```python
from build123d import *

# Parameters (mm, degrees)
BOSS_EXTRUDE1_DEPTH   = 3.175
SKETCH2_W             = 12.7
SKETCH2_H             = 12.7
BOSS_EXTRUDE2_DEPTH   = 28.575
SKETCH3_R             = 2.5
CUT_EXTRUDE1_DEPTH    = 10
CHAMFER1_SIZE         = 12.7
CHAMFER1_SIZE2        = 7.332348419
CHAMFER1_PART_2_SIZE  = 12.7
CHAMFER1_PART_2_SIZE2 = 7.332348419
CHAMFER1_PART_3_SIZE  = 12.7
CHAMFER1_PART_3_SIZE2 = 7.332348419
FILLET1_R             = 3.175
FILLET2_R             = 3.175
FILLET4_R             = 1.5875


with BuildPart() as part:
    # Sketch1 → Boss-Extrude1 (new body)
    with BuildSketch(Plane.XY):
        Polygon((38.1, 0), (-38.1, 0), (-38.1, -12.7), (-19.05, -12.7), (-19.05, -69.85), (-6.35, -69.85), (-6.35, -38.1), (19.05, -12.7), (38.1, -12.7), align=None)
    extrude(amount=BOSS_EXTRUDE1_DEPTH)

    # Sketch2 → Boss-Extrude2 (add)
    with BuildSketch(Plane(origin=(0, 0, 0), x_dir=(-1, 0, 0), z_dir=(0, 0, -1))):
        with Locations((-31.75, -6.35)):
            Rectangle(SKETCH2_W, SKETCH2_H)
        with Locations((31.75, -6.35)):
            Rectangle(SKETCH2_W, SKETCH2_H)
        with Locations((12.7, -63.5)):
            Rectangle(SKETCH2_W, SKETCH2_H)
    extrude(amount=BOSS_EXTRUDE2_DEPTH)

    # Sketch3 → Cut-Extrude1 (cut)
    with BuildSketch(Plane(origin=(0, 0, -28.575), x_dir=(-1, 0, 0), z_dir=(0, 0, -1))):
        with Locations((-31.75, -6.35)):
            Circle(SKETCH3_R)
        with Locations((31.75, -6.35)):
            Circle(SKETCH3_R)
        with Locations((12.7, -63.5)):
            Circle(SKETCH3_R)
    extrude(amount=-CUT_EXTRUDE1_DEPTH, mode=Mode.SUBTRACT)

    # Chamfer1
    chamfer1_edges = [part.edges().sort_by_distance(p)[0] for p in [
        (38.1, -6.35, 3.175),
    ]]
    chamfer1_side = [part.faces().sort_by_distance(p)[0] for p in [
        (38.1, -6.35, -12.7),
    ]]
    chamfer(chamfer1_edges, length=CHAMFER1_SIZE, length2=CHAMFER1_SIZE2, reference=chamfer1_side[0])

    # Chamfer1 part 2
    chamfer1_part_2_edges = [part.edges().sort_by_distance(p)[0] for p in [
        (-38.1, -6.35, 3.175),
    ]]
    chamfer1_part_2_side = [part.faces().sort_by_distance(p)[0] for p in [
        (-38.1, -6.35, -12.7),
    ]]
    chamfer(chamfer1_part_2_edges, length=CHAMFER1_PART_2_SIZE, length2=CHAMFER1_PART_2_SIZE2, reference=chamfer1_part_2_side[0])

    # Chamfer1 part 3
    chamfer1_part_3_edges = [part.edges().sort_by_distance(p)[0] for p in [
        (-12.7, -69.85, 3.175),
    ]]
    chamfer1_part_3_side = [part.faces().sort_by_distance(p)[0] for p in [
        (-12.7, -69.85, -12.7),
    ]]
    chamfer(chamfer1_part_3_edges, length=CHAMFER1_PART_3_SIZE, length2=CHAMFER1_PART_3_SIZE2, reference=chamfer1_part_3_side[0])

    # Fillet1
    fillet1_edges = [part.edges().sort_by_distance(p)[0] for p in [
        (-6.35, -38.1, 1.5875),
        (-19.05, -12.7, 1.5875),
        (19.05, -12.7, 1.5875),
    ]]
    fillet(fillet1_edges, radius=FILLET1_R)

    # Fillet2
    fillet2_edges = [part.edges().sort_by_distance(p)[0] for p in [
        (25.4, -12.7, -14.2875),
        (25.4, 0, -14.2875),
        (-25.4, 0, -14.2875),
        (-25.4, -12.7, -14.2875),
        (-19.05, -57.15, -14.2875),
        (-6.35, -57.15, -14.2875),
        (38.1, 0, -19.05),
        (-38.1, 0, -19.05),
        (38.1, -12.7, -19.05),
        (-6.35, -69.85, -19.05),
        (-19.05, -69.85, -19.05),
        (-38.1, -12.7, -19.05),
    ]]
    fillet(fillet2_edges, radius=FILLET2_R)

    # Fillet4
    fillet4_edges = [part.edges().sort_by_distance(p)[0] for p in [
        (-12.7, -57.15, -28.575),
        (-19.05, -63.5, -28.575),
        (-6.35, -63.5, -28.575),
        (-12.7, -69.85, -28.575),
        (-7.27993597, -58.07993597, -28.575),
        (-7.27993597, -68.92006403, -28.575),
        (-18.12006403, -68.92006403, -28.575),
        (-18.12006403, -58.07993597, -28.575),
        (38.1, -6.35, -28.575),
        (31.75, -12.7, -28.575),
        (25.4, -6.35, -28.575),
        (31.75, 0, -28.575),
        (26.32993597, -11.77006403, -28.575),
        (26.32993597, -0.92993597, -28.575),
        (37.17006403, -0.92993597, -28.575),
        (37.17006403, -11.77006403, -28.575),
        (-31.75, 0, -28.575),
        (-25.4, -6.35, -28.575),
        (-38.1, -6.35, -28.575),
        (-31.75, -12.7, -28.575),
        (-37.17006403, -11.77006403, -28.575),
        (-37.17006403, -0.92993597, -28.575),
        (-26.32993597, -11.77006403, -28.575),
        (-26.32993597, -0.92993597, -28.575),
    ]]
    fillet(fillet4_edges, radius=FILLET4_R)


solid = part.part
```
Part model, mm, in its own coordinate system. A direction names the side the tool comes from. Give positions to 0.01 mm unless a question says otherwise; leave off trailing zeros. Write each loop counter-clockwise with the first axis right and the second up, starting at its lowest first coordinate (ties: lowest second). Pieces come first, ordered by that corner, then holes. Notation, with made-up numbers: (43.5, 30) -> (86.5, 30) arc R29 cw to (86.5, 61) -> close; hole circle Ø10 at (13.5, -1). An arc over 180 degrees is marked (long way). Put each result on its own line as item: value. Start each with the question number.
Item 1: Pin check, flat tips, straight feed: pin 1 Ø1.9 at (x, z) = (-11, -8) entering from +Y; pin 2 Ø13.5 at (y, z) = (-51.5, -5.5) entering from +X; pin 3 Ø1 at (x, z) = (28, -0.5) entering from -Y. Stop position of each tip, or through.
Item 2: Cut at A-A (z = -11.5). List the corners of the cut face in (x, y) (3 decimals), then the cut area to 3 significant figures.
Item 3: Which spindle directions (+Z, -Z, +X, -X, +Y, -Y) get a long thin tool onto all of the face, cutting with end or side? Do faces 5 (the face through (-32, -6, -18.575)), 6 (the face through (-18.14, -58.1, -13.68)), 7 (the face through (-31, -12.7, -12)), 8 (the face through (31, -12.7, -12)). Say none if no direction does.
Item 4: Wall check: L1, parallel to Y at x = 31.75, z = -25.75; L2, parallel to Y at x = -12.7, z = -23; L3, parallel to Y at x = -29.5, z = -15.5. Give the ranges that are in metal, low to high. Write a range as [from, to].
Item 5: Pull direction X, two halves, no side cores. Call faces 1 (the face through (-34.06, -7.31, -23.64)), 2 (the face through (-25.4, -6, -13)), 3 (the face through (-6.35, -61, -10)), 4 (the face through (-19.05, -48.7, 0.3)): pulls with the +X half, pulls with the -X half, needs draft (parallel to the pull), parting line crosses it, or undercut.
Item 6: Cut at D-D (z = -3). List the corners of the cut face in (x, y) (3 decimals), then the cut area to 3 significant figures.
Answer list:
1. pin 1: stops at y = -57.15
1. pin 2: stops at x = -6.35
1. pin 3: stops at y = -12.7
2. outline: (-38.1, -9.525) arc R3.175 ccw to (-34.925, -12.7) -> (-28.575, -12.7) arc R3.175 ccw to (-25.4, -9.525) -> (-25.4, -3.175) arc R3.175 ccw to (-28.575, 0) -> (-34.925, 0) arc R3.175 ccw to (-38.1, -3.175) -> close; (-19.05, -66.675) arc R3.175 ccw to (-15.875, -69.85) -> (-9.525, -69.85) arc R3.175 ccw to (-6.35, -66.675) -> (-6.35, -60.325) arc R3.175 ccw to (-9.525, -57.15) -> (-15.875, -57.15) arc R3.175 ccw to (-19.05, -60.325) -> close; (25.4, -9.525) arc R3.175 ccw to (28.575, -12.7) -> (34.925, -12.7) arc R3.175 ccw to (38.1, -9.525) -> (38.1, -3.175) arc R3.175 ccw to (34.925, 0) -> (28.575, 0) arc R3.175 ccw to (25.4, -3.175) -> close
2. area: 458 mm2
3. face 5: -Z
3. face 6: -Z, -X, +Y
3. face 7: +Z, -Z, -X, -Y
3. face 8: +Z, -Z, +X, -Y
4. L1: y = [-12.7, -8.85], [-3.85, 0]
4. L2: y = [-69.85, -66], [-61, -57.15]
4. L3: y = [-12.7, 0]
5. face 1: undercut
5. face 2: undercut
5. face 3: pulls with the +X half
5. face 4: pulls with the -X half
6. outline: (-34.333, -12.7) -> (-28.575, -12.7) arc R3.175 ccw to (-25.4, -9.525) -> (-25.4, -3.175) arc R3.175 ccw to (-28.575, 0) -> (-34.333, 0) -> close; (-19.05, -66.083) -> (-6.35, -66.083) -> (-6.35, -60.325) arc R3.175 ccw to (-9.525, -57.15) -> (-15.875, -57.15) arc R3.175 ccw to (-19.05, -60.325) -> close; (25.4, -9.525) arc R3.175 ccw to (28.575, -12.7) -> (34.333, -12.7) -> (34.333, 0) -> (28.575, 0) arc R3.175 ccw to (25.4, -3.175) -> close
6. area: 327 mm2
